Here's how the part is built. I have some questions about the finished solid (model axes, mm). Give positions to 0.01 mm unless a question says otherwise; leave off trailing zeros. Write each loop counter-clockwise with the first axis right and the second up, starting at its lowest first coordinate (ties: lowest second). Pieces come first, ordered by that corner, then holes. Notation, with made-up numbers: (20.5, 86.25) -> (50.5, 86.25) arc R26 cw to (50.5, 102.25) -> close; hole circle Ø2 at (67.5, -33.75). An arc over 180 degrees is marked (long way). Use CSV: the item, a comma, the result in double quotes. Start each with the question number.
(1) Suppose I cut it at B-B on z = 3.8. List the corners of the cut face in (x, y) for me, plus the area to 3 significant figures.
(2) Suppose I cut it at C-C on y = 2.95. List the corners of the cut face in (x, z) for me.
(3) Suppose I cut it at A-A on x = -27.5. List the corners of the cut face in (y, z) for me.
(4) I need wall thicknesses on L1, parallel to Y at x = -22.75, z = 3.15; L2, parallel to Z at x = -30, y = 3.2; L3, parallel to Y at x = -18.75, z = 3.7. Which ranges of each line are inside material? Lowest first, please. Write a range as [from, to].
from build123d import *

# Parameters (mm, degrees)
BOX006_W     = 17
BOX006_H     = 2
BOX006_DEPTH = 1
FILLET008_R  = 0.9
FILLET009_R  = 0.9


with BuildPart() as part:
    # Box006 → Box006 (new body)
    with BuildSketch(Plane(origin=(-31, -4.75, 3), x_dir=(1, 0, 0), z_dir=(0, 0, 1))):
        with Locations((8.5, 1)):
            Rectangle(BOX006_W, BOX006_H)
    extrude(amount=BOX006_DEPTH)

    # Fillet008
    fillet008_edges = [part.edges().sort_by_distance(p)[0] for p in [
        (-22.5, -4.75, 4),
    ]]
    fillet(fillet008_edges, radius=FILLET008_R)

    # Fillet009
    fillet009_edges = [part.edges().sort_by_distance(p)[0] for p in [
        (-22.5, -2.75, 4),
    ]]
    fillet(fillet009_edges, radius=FILLET009_R)


with BuildPart() as part_1:
    # Fillet009 placement: moved
    add(part.part.moved(Location((0, 7.5, 0))))


solid = part_1.part
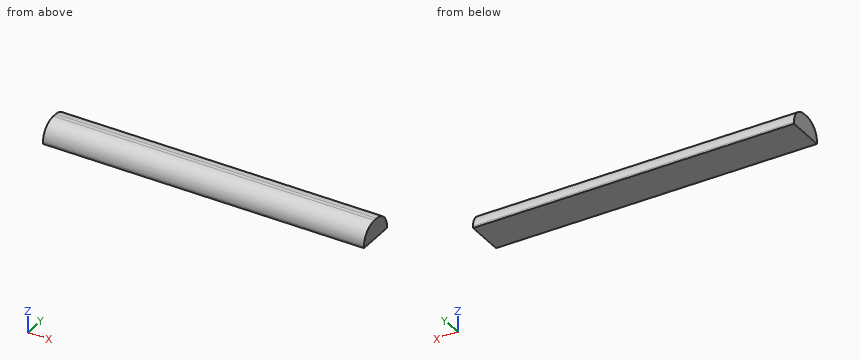
Geometry says:
1,outline,"(-31, 3.08) -> (-14, 3.08) -> (-14, 4.42) -> (-31, 4.42) -> close"
1,area,"22.6 mm²"
2,outline,"(-31, 3) -> (-14, 3) -> (-14, 3.67) -> (-31, 3.67) -> close"
3,outline,"(2.75, 3) -> (4.75, 3) -> (4.75, 3.1) arc R0.9 ccw to (3.85, 4) -> (3.65, 4) arc R0.9 ccw to (2.75, 3.1) -> close"
4,L1,"[2.75, 4.75]"
4,L2,"[3, 3.88]"
4,L3,"[2.98, 4.52]"
